Source: CAD feature listing. Evaluate the final solid. Frame: model axes, mm. A direction names the side the tool comes from. Coordinates: 2 decimals unless noted, no trailing zeros. Write each loop counter-clockwise with the first axis right and the second up, starting at its lowest first coordinate (ties: lowest second). Pieces come first, ordered by that corner, then holes. Notation, with made-up numbers: M 16,-20.75 L 29,-20.75 A21 ccw 29,13.25 Z; hole C -24.5,85 d7. An arc over 180 degrees is marked long. One line per item, written item: value. Start each with the question number.
Item 1: Set-up query: faces 1 (the flat face through (-50, 27, 3)), 2 (the flat face through (50, 28, 3)), 3 (the flat face through (-53, -10, 3)). Return all of +Z, -Z, +X, -X, +Y, -Y with unobstructed straight access to the full face (end or side cutting, diameter ignored); none if empty.
Item 2: Pin query (flat end, axial travel): P1, Ø2, axis at x = 54, z = 4.5, coming from the +Y side; P2, Ø1.2, axis at x = -54, z = 3, coming from the -Y side; P3, Ø1.2, axis at y = -47.5, z = 4, coming from the -X side. Return the tip coordinate at first contact, or that it passes through.
Item 3: Ray query, L1, parallel to X at y = 37.5, z = 5.55; L2, parallel to Y at x = -34.5, z = 0.85. Return the intervals inside material, ascending. Write a range as from..to.
Item 4: Cut plane B-B, the plane y = -41. Output: boundary loops of the cut face in (x, z).
Item 5: Cut plane A-A, the plane x = -25.5. Output: boundary loops of the cut face in (y, z), then the cut area to 3 significant figures.
```python
from build123d import *

# Parameters (mm, degrees)
BOSS_EXTRUDE1_DEPTH = 6
FILLET1_R           = 1


with BuildPart() as part:
    # Sketch1 → Boss-Extrude1 (new body)
    with BuildSketch(Plane.XY):
        Polygon((50, 10), (56, 10), (56, -10), (50, -10), (50, -44), (10, -44), (10, -50), (-10, -50), (-10, -44), (-50, -44), (-50, -10), (-56, -10), (-56, 10), (-50, 10), (-50, 44), (-10, 44), (-10, 50), (10, 50), (10, 44), (50, 44), align=None)
    extrude(amount=BOSS_EXTRUDE1_DEPTH)

    # Fillet1
    fillet1_edges = [part.edges().sort_by_distance(p)[0] for p in [
        (10, -44, 3),
        (10, -50, 3),
        (-10, -50, 3),
        (-10, -44, 3),
        (-50, -10, 3),
        (-56, -10, 3),
        (-56, 10, 3),
        (-50, 10, 3),
        (-10, 44, 3),
        (-10, 50, 3),
        (10, 50, 3),
        (10, 44, 3),
        (50, 10, 3),
        (56, 10, 3),
        (56, -10, 3),
        (50, -10, 3),
    ]]
    fillet(fillet1_edges, radius=FILLET1_R)


solid = part.part
```
From the geometry:
1. face 1: +Z, -Z, -X, +Y
1. face 2: +Z, -Z, +X, +Y
1. face 3: +Z, -Z, -X, -Y
2. P1: stops at y = 10
2. P2: stops at y = -10
2. P3: stops at x = -10
3. L1: x = -50..50
3. L2: y = -44..44
4. outline: M -50,0 L 50,0 L 50,6 L -50,6 Z
5. outline: M -44,0 L 44,0 L 44,6 L -44,6 Z
5. area: 528 mm²
